from build123d import *

# Parameters (mm, degrees)
SKETCH_1_R          = 32.5
EXTRUDE_1_DEPTH     = 10
SKETCH_2_R          = 67.5
EXTRUDE_2_DEPTH     = 12
SKETCH_3_R          = 19
CUT_EXTRUDE_1_DEPTH = 45
SKETCH_4_R          = 32.5
SKETCH_4_R_2        = 19
EXTRUDE_3_DEPTH     = 33
SKETCH_5_W          = 10
SKETCH_5_H          = 9.79155849
CUT_EXTRUDE_2_DEPTH = 111.170322683
SKETCH_6_R          = 4
CUT_EXTRUDE_3_DEPTH = 30
CHAMFER_1_SIZE      = 1
CHAMFER_2_SIZE      = 0.5
CHAMFER_3_SIZE      = 2
CHAMFER_4_SIZE      = 1


with BuildPart() as part:
    # 草图1 → 拉伸1 (new body)
    with BuildSketch(Plane.XY):
        Circle(SKETCH_1_R)
    extrude(amount=EXTRUDE_1_DEPTH)

    # 草图2 → 拉伸2 (add)
    with BuildSketch(Plane.XY.offset(10)):
        Circle(SKETCH_2_R)
    extrude(amount=EXTRUDE_2_DEPTH)

    # 草图3 → 切除-拉伸1 (cut)
    with BuildSketch(Plane.XY.offset(22)):
        Circle(SKETCH_3_R)
    extrude(amount=-CUT_EXTRUDE_1_DEPTH, mode=Mode.SUBTRACT)

    # 草图4 → 拉伸3 (add)
    with BuildSketch(Plane.XY.offset(22)):
        Circle(SKETCH_4_R)
        Circle(SKETCH_4_R_2, mode=Mode.SUBTRACT)
    extrude(amount=EXTRUDE_3_DEPTH)

    # 草图5 → 切除-拉伸2 (cut, through all)
    with BuildSketch(Plane(origin=(0, 0, 0), x_dir=(-1, 0, 0), z_dir=(0, 0, -1))):
        with Locations((0, 17.104220755)):
            Rectangle(SKETCH_5_W, SKETCH_5_H)
    extrude(amount=-CUT_EXTRUDE_2_DEPTH, mode=Mode.SUBTRACT)

    # 草图6 → 切除-拉伸3 (cut)
    with BuildSketch(Plane.XY.offset(22)):
        with Locations((40.658639918, 40.658639918)):
            Circle(SKETCH_6_R)
        with Locations((0, 57.5)):
            Circle(SKETCH_6_R)
        with Locations((57.5, 0)):
            Circle(SKETCH_6_R)
        with Locations((40.658639918, -40.658639918)):
            Circle(SKETCH_6_R)
        with Locations((0, -57.5)):
            Circle(SKETCH_6_R)
        with Locations((-40.658639918, -40.658639918)):
            Circle(SKETCH_6_R)
        with Locations((-57.5, 0)):
            Circle(SKETCH_6_R)
        with Locations((-40.658639918, 40.658639918)):
            Circle(SKETCH_6_R)
    extrude(amount=-CUT_EXTRUDE_3_DEPTH, mode=Mode.SUBTRACT)

    # 倒角1
    chamfer_1_edges = [part.edges().sort_by_distance(p)[0] for p in [
        (-32.5, 0, 55),
        (-32.5, 0, 0),
        (0, -19, 55),
        (-67.5, 0, 10),
    ]]
    chamfer(chamfer_1_edges, length=CHAMFER_1_SIZE)

    # 倒角2
    chamfer_2_edges = [part.edges().sort_by_distance(p)[0] for p in [
        (-4, 57.5, 10),
        (-4, 57.5, 22),
        (36.658639918, 40.658639918, 10),
        (36.658639918, 40.658639918, 22),
        (53.5, 0, 10),
        (53.5, 0, 22),
        (36.658639918, -40.658639918, 10),
        (36.658639918, -40.658639918, 22),
        (-4, -57.5, 10),
        (-4, -57.5, 22),
        (-44.658639918, -40.658639918, 10),
        (-44.658639918, -40.658639918, 22),
        (-61.5, 0, 10),
        (-61.5, 0, 22),
        (-44.658639918, 40.658639918, 10),
        (-44.658639918, 40.658639918, 22),
    ]]
    chamfer(chamfer_2_edges, length=CHAMFER_2_SIZE)

    # 倒角3
    chamfer_3_edges = [part.edges().sort_by_distance(p)[0] for p in [
        (-67.5, 0, 22),
    ]]
    chamfer(chamfer_3_edges, length=CHAMFER_3_SIZE)

    # 倒角4
    chamfer_4_edges = [part.edges().sort_by_distance(p)[0] for p in [
        (0, -19, 0),
    ]]
    chamfer(chamfer_4_edges, length=CHAMFER_4_SIZE)


solid = part.part
Can you work these out from the model? Positions are in its coordinate system, mm. A direction names the side the tool comes from. Round coordinates to 2 decimals unless told otherwise and drop trailing zeros. Loops run counter-clockwise (first coordinate to the right, second up) from the corner with the lowest first, then second, coordinate; pieces in that order, holes last. Notation, with made-up numbers: (51.25, 19.25) - (95.25, 19.25) arc R22 cw to (95.25, 49.25) - close; hole circle Ø1 at (86, 82.5). An arc over 180 degrees is marked (long way). Answer in a Markdown table with one row per item. Add a question column.
Q1. We'd pull the mould along Y, two halves only. Please class faces 4 (the conical face through (-8.54, 65.07, 21.87)), 5 (the cylindrical face through (61.315, 1.201, 16.077)): pulls with the +Y half, pulls with the -Y half, needs draft (parallel to the pull), parting line crosses it, or undercut.
Q2. For pin 1 Ø23 at (x, y) = (0, 0) entering from +Z (3 decimals); pin 2 Ø13 at (x, y) = (40.66, 40.66) entering from +Z; pin 3 Ø4 at (y, z) = (20.5, 39.5) entering from +X; pin 4 Ø1.5 at (y, z) = (-9, 18.5) entering from -X, each with a flat end and sliding along its axis, tell me the tip position at first contact or that it passes through.
Q3. I need wall thicknesses on L1, parallel to Y at x = 0, z = 17; L2, parallel to X at y = 57, z = 15; L3, parallel to Y at x = 0, z = 27. Which ranges of each line are inside material? Lowest first, please.
Q4. I want a section at A-A on z = 5.5. List the corners of the cut face in (x, y) for me, and give its area (3 significant figures).
Q5. I want a section at B-B on y = 0. Count the separate pieces of the cut face and the enclosed holes in it, and give its area (3 significant figures).
Q6. Which directions (+Z, -Z, +X, -X, +Y, -Y) give clear straight access to the entire face, cutting with the end or side of a thin tool? Please do faces 1 (the cylindrical face through (31, 9.76, 5.44)), 2 (the flat face through (0, 22, 27)), 3 (the cylindrical face through (31, 9.76, 37.78)).
A:
| question | item | result |
|---|---|---|
| 1 | face 4 | parting line crosses it |
| 1 | face 5 | undercut |
| 2 | pin 1 | through |
| 2 | pin 2 | z = 22 |
| 2 | pin 3 | x = 26.72 |
| 2 | pin 4 | x = -66.99 |
| 3 | L1 | -67.5 to -61.5, -53.5 to -19, 22 to 53.5, 61.5 to 67.5 |
| 3 | L2 | -36.16 to -3.97, 3.97 to 36.16 |
| 3 | L3 | -32.5 to -19, 22 to 32.5 |
| 4 | outline | circle Ø65 at (0, 0); hole (-5, 18.33) arc R19 ccw (long way) to (5, 18.33) - (5, 22) - (-5, 22) - close |
| 4 | area | 2,150 mm^2 |
| 5 | separate pieces | 4 |
| 5 | enclosed holes | 0 |
| 5 | area | 2,120 mm^2 |
| 6 | face 1 | -Z |
| 6 | face 2 | +Z, -Z |
| 6 | face 3 | +Z |
